```python
from build123d import *
from OCP.BRepFilletAPI import BRepFilletAPI_MakeChamfer

# Parameters (mm, degrees)
CROQUIS1_W              = 226.5
CROQUIS1_H              = 226.9
CROQUIS1_R              = 18.85
CROQUIS1_R_2            = 5.05
CROQUIS1_R_3            = 2.6
SALIENTE_EXTRUIR1_DEPTH = 10
CHAFL_N1_SIZE           = 10
CHAFL_N1_SIZE_2         = 6.7
CROQUIS5_R              = 34.95
CROQUIS5_R_2            = 18.85
SALIENTE_EXTRUIR7_DEPTH = 21.2


with BuildPart() as part:
    # Croquis1 → Saliente-Extruir1 (new body)
    with BuildSketch(Plane(origin=(0, 0, 0), x_dir=(1, 0, 0), z_dir=(0, 1, 0))):
        Rectangle(CROQUIS1_W, CROQUIS1_H)
        with Locations(Location((0, 0, 0), (0, 0, 270))):
            Circle(CROQUIS1_R, mode=Mode.SUBTRACT)
        with Locations(Location((-101.5, 0, 0), (0, 0, 270))):
            Circle(CROQUIS1_R_2, mode=Mode.SUBTRACT)
        with Locations(Location((-101.5, -25.4, 0), (0, 0, 270))):
            Circle(CROQUIS1_R_3, mode=Mode.SUBTRACT)
        with Locations(Location((-101.5, -50.85, 0), (0, 0, 270))):
            Circle(CROQUIS1_R_3, mode=Mode.SUBTRACT)
        with Locations(Location((-101.5, -76.3, 0), (0, 0, 270))):
            Circle(CROQUIS1_R_3, mode=Mode.SUBTRACT)
        with Locations(Location((-101.5, -101.7, 0), (0, 0, 270))):
            Circle(CROQUIS1_R_2, mode=Mode.SUBTRACT)
        with Locations(Location((-101.5, 101.7, 0), (0, 0, 90))):
            Circle(CROQUIS1_R_2, mode=Mode.SUBTRACT)
        with Locations(Location((-101.5, 76.3, 0), (0, 0, 90))):
            Circle(CROQUIS1_R_3, mode=Mode.SUBTRACT)
        with Locations(Location((-101.5, 50.85, 0), (0, 0, 90))):
            Circle(CROQUIS1_R_3, mode=Mode.SUBTRACT)
        with Locations(Location((-101.5, 25.4, 0), (0, 0, 90))):
            Circle(CROQUIS1_R_3, mode=Mode.SUBTRACT)
        with Locations(Location((101.5, -101.7, 0), (0, 0, 90))):
            Circle(CROQUIS1_R_2, mode=Mode.SUBTRACT)
        with Locations(Location((101.5, -76.3, 0), (0, 0, 90))):
            Circle(CROQUIS1_R_3, mode=Mode.SUBTRACT)
        with Locations(Location((101.5, -50.85, 0), (0, 0, 90))):
            Circle(CROQUIS1_R_3, mode=Mode.SUBTRACT)
        with Locations(Location((101.5, -25.4, 0), (0, 0, 90))):
            Circle(CROQUIS1_R_3, mode=Mode.SUBTRACT)
        with Locations(Location((101.5, 0, 0), (0, 0, 90))):
            Circle(CROQUIS1_R_2, mode=Mode.SUBTRACT)
        with Locations(Location((101.5, 25.4, 0), (0, 0, 270))):
            Circle(CROQUIS1_R_3, mode=Mode.SUBTRACT)
        with Locations(Location((101.5, 50.85, 0), (0, 0, 270))):
            Circle(CROQUIS1_R_3, mode=Mode.SUBTRACT)
        with Locations(Location((101.5, 76.3, 0), (0, 0, 270))):
            Circle(CROQUIS1_R_3, mode=Mode.SUBTRACT)
        with Locations(Location((101.5, 101.7, 0), (0, 0, 270))):
            Circle(CROQUIS1_R_2, mode=Mode.SUBTRACT)
        with Locations(Location((76.499655125, 101.349606639, 0), (0, 0, 90))):
            Circle(CROQUIS1_R_3, mode=Mode.SUBTRACT)
        with Locations(Location((51.049704434, 101.399705015, 0), (0, 0, 90))):
            Circle(CROQUIS1_R_3, mode=Mode.SUBTRACT)
        with Locations(Location((25.599753743, 101.449803392, 0), (0, 0, 90))):
            Circle(CROQUIS1_R_3, mode=Mode.SUBTRACT)
        with Locations(Location((0.199802956, 101.499803344, 0), (0, 0, 90))):
            Circle(CROQUIS1_R_2, mode=Mode.SUBTRACT)
        with Locations(Location((-25.200147831, 101.549803295, 0), (0, 0, 270))):
            Circle(CROQUIS1_R_3, mode=Mode.SUBTRACT)
        with Locations(Location((-50.650098522, 101.599901672, 0), (0, 0, 270))):
            Circle(CROQUIS1_R_3, mode=Mode.SUBTRACT)
        with Locations(Location((-76.100049213, 101.650000048, 0), (0, 0, 270))):
            Circle(CROQUIS1_R_3, mode=Mode.SUBTRACT)
        with Locations(Location((76.499655125, -101.349606639, 0), (0, 0, 270))):
            Circle(CROQUIS1_R_3, mode=Mode.SUBTRACT)
        with Locations(Location((51.049704434, -101.399705015, 0), (0, 0, 270))):
            Circle(CROQUIS1_R_3, mode=Mode.SUBTRACT)
        with Locations(Location((25.599753743, -101.449803392, 0), (0, 0, 270))):
            Circle(CROQUIS1_R_3, mode=Mode.SUBTRACT)
        with Locations(Location((0.199802956, -101.499803344, 0), (0, 0, 270))):
            Circle(CROQUIS1_R_2, mode=Mode.SUBTRACT)
        with Locations(Location((-25.200147831, -101.549803295, 0), (0, 0, 90))):
            Circle(CROQUIS1_R_3, mode=Mode.SUBTRACT)
        with Locations(Location((-50.650098522, -101.599901672, 0), (0, 0, 90))):
            Circle(CROQUIS1_R_3, mode=Mode.SUBTRACT)
        with Locations(Location((-76.100049213, -101.650000048, 0), (0, 0, 90))):
            Circle(CROQUIS1_R_3, mode=Mode.SUBTRACT)
    extrude(amount=SALIENTE_EXTRUIR1_DEPTH)

    # Chaflán1
    chafl_n1_edges_1 = [part.edges().sort_by_distance(p)[0] for p in [
        (0, 10, -113.45),
    ]]
    chafl_n1_side_1 = [part.faces().sort_by_distance(p)[0] for p in [
        (0, 9.866, -113.45),
    ]]
    chafl_n1_edges_2 = [part.edges().sort_by_distance(p)[0] for p in [
        (113.25, 10, 0),
    ]]
    chafl_n1_side_2 = [part.faces().sort_by_distance(p)[0] for p in [
        (113.25, 9.866, 0),
    ]]
    chafl_n1_edges_3 = [part.edges().sort_by_distance(p)[0] for p in [
        (0, 10, 113.45),
    ]]
    chafl_n1_side_3 = [part.faces().sort_by_distance(p)[0] for p in [
        (0, 9.866, 113.45),
    ]]
    chafl_n1_edges_4 = [part.edges().sort_by_distance(p)[0] for p in [
        (-113.25, 10, 0),
    ]]
    chafl_n1_side_4 = [part.faces().sort_by_distance(p)[0] for p in [
        (-113.25, 9.866, 0),
    ]]
    chafl_n1 = BRepFilletAPI_MakeChamfer(part.part.solid().wrapped)
    for e in chafl_n1_edges_1:
        chafl_n1.Add(CHAFL_N1_SIZE - 0.0001, CHAFL_N1_SIZE_2 - 0.0001, e.wrapped, chafl_n1_side_1[0].wrapped)
    for e in chafl_n1_edges_2:
        chafl_n1.Add(CHAFL_N1_SIZE - 0.0001, CHAFL_N1_SIZE_2 - 0.0001, e.wrapped, chafl_n1_side_2[0].wrapped)
    for e in chafl_n1_edges_3:
        chafl_n1.Add(CHAFL_N1_SIZE - 0.0001, CHAFL_N1_SIZE_2 - 0.0001, e.wrapped, chafl_n1_side_3[0].wrapped)
    for e in chafl_n1_edges_4:
        chafl_n1.Add(CHAFL_N1_SIZE - 0.0001, CHAFL_N1_SIZE_2 - 0.0001, e.wrapped, chafl_n1_side_4[0].wrapped)
    add(Compound.cast(chafl_n1.Shape()), mode=Mode.REPLACE)  # a hair under: the kernel refuses the full size

    # Croquis5 → Saliente-Extruir7 (add)
    with BuildSketch(Plane(origin=(0, 10, 0), x_dir=(1, 0, 0), z_dir=(0, 1, 0))):
        with Locations(Location((0, 0, 0), (0, 0, 270))):
            Circle(CROQUIS5_R)
        with Locations(Location((0, 0, 0), (0, 0, 270))):
            Circle(CROQUIS5_R_2, mode=Mode.SUBTRACT)
    extrude(amount=SALIENTE_EXTRUIR7_DEPTH)


solid = part.part
```
Input: part model. Units: mm. Frame: model coordinates. A direction names the side the tool comes from. Give positions to 0.01 mm unless a question says otherwise; leave off trailing zeros.
1. Pin query (flat end, axial travel): pin 1 Ø6 at (x, z) = (101.5, 76.3) entering from +Y; pin 2 Ø5 at (x, y) = (-21.5, 8) entering from -Z; pin 3 Ø10 at (y, z) = (10.5, 83) entering from -X. Return the tip coordinate at first contact, or that it passes through.
Computed:
pin 1: stops at y = 10
pin 2: stops at z = -109.77
pin 3: stops at x = -109.57
2. Cut plane A-A (z = 0). State how many separate pieces and enclosed holes the cut face has, and give its area (3 significant figures).
Computed:
separate pieces: 4
enclosed holes: 0
area: 2,300 mm2
3. Line query: probe 1 along X at (y, z) = (5, -25.4); probe 2 along Y at (x, z) = (65.5, -36); probe 3 along Z at (x, y) = (-52.5, 8). Output: solid intervals per line, ascending.
Computed:
probe 1: x = -109.9 to -104.1, -98.9 to 98.9, 104.1 to 109.9
probe 2: y = 0 to 10
probe 3: z = -108.09 to -103.43, -99.77 to 99.77, 103.43 to 108.09
4. Draft query along X for faces 1 (the face through (-1.585, 5.07, -110.053)), 2 (the face through (109.853, 5.07, 1.588)), 3 (the face through (-104.913, 4.93, -97.978)). Return one class per face: released by +X, released by -X, zero draft, split by the parting line, or undercut.
Computed:
face 1: zero draft
face 2: released by +X
face 3: undercut
5. Set-up query: faces 4 (the face through (10.498, 20.452, 33.336)), 5 (the face through (-98.087, 4.93, 97.978)). Return all of +Z, -Z, +X, -X, +Y, -Y with unobstructed straight access to the full face (end or side cutting, diameter ignored); none if empty.
Computed:
face 4: +Y
face 5: +Y, -Y
